Here's how the part is built. I have some questions about the finished solid (model axes, mm). A direction names the side the tool comes from. Give positions to 0.01 mm unless a question says otherwise; leave off trailing zeros. Write each loop counter-clockwise with the first axis right and the second up, starting at its lowest first coordinate (ties: lowest second). Pieces come first, ordered by that corner, then holes. Notation, with made-up numbers: M 88.25,-18.5 L 121.25,-18.5 A19 ccw 121.25,-3.5 Z; hole C 73.5,-33 d5. An arc over 180 degrees is marked long. Answer as CSV lines item,"result". Start each with the question number.
Q1. Suppose I cut it at C-C (x = -37). Write out the boundary of the cut face in (y, z).
Q2. For pin 1 (4 mm diameter, centred on x = -14.5, z = -57.5, fed in from -Y), with a flat end and sliding along its axis, tell me the tip position at first contact or that it passes through.
Q3. Thinking about a two-plate mould opening in Z: for faces 3 (the flat face through (-38, 10, -75)), 4 (the cylindrical face through (-26.508, 10.14, -40.304)), 5 (the flat face through (0, 10, -38)), which applies, +Z half, -Z half, draft (parallel to the pull), parting line (faces both ways), or undercut?
Q4. Suppose I cut it at B-B (z = -37). Write out the boundary of the cut face in (x, y).
Q5. On a 3-axis mill with a long thin cutter (end or side, diameter ignored), from which of +Z, -Z, +X, -X, +Y, -Y can I reach the whole of each face in a straight line? I mean faces 1 (the flat face through (-37, 10, 0)), 2 (the flat face through (-37, 7, -5)). Say none if no direction works.
Q6. If I drill on line 1 along Z through (x, y) = (-37, 8.5); line 2 along Z through (x, y) = (-18.5, 2), over which ranges is the centre line in solid material (lowest first)?
Q7. Suppose I cut it at A-A (y = 9.5). Write out the boundary of the cut face in (x, z), then the cut area to 3 significant figures.
Q8. Suppose I cut it at D-D (x = -64.5). Write out the boundary of the cut face in (y, z).
Autodesk Inventor part; units mm, degrees
ref_plane "YZ Plane" through (0, 0, 0) normal (1, 0, 0) x (0, 1, 0)
ref_plane "XZ Plane" through (0, 0, 0) normal (0, 1, 0) x (-1, 0, 0)
ref_plane "XY Plane" through (0, 0, 0) normal (0, 0, 1) x (1, 0, 0)
sketch "Sketch1" plane through (0, 0, 0) normal (0, 1, 0) x (-1, 0, 0)
  point P0 (0, 0)
sketch "Sketch2" plane through (0, 0, 0) normal (0, 1, 0) x (-1, 0, 0)
  line L0 (0, 0) -> (75, 0)
  line L1 (75, 0) -> (75, -75)
  line L2 (75, -75) -> (0, -75)
  line L3 (0, -75) -> (0, 0)
  dimension "d0" = 75
  dimension "d1" = 75
extrude "Extrusion1" add sketch "Sketch2" along normal blind 20
sketch "Sketch3" plane through (0, 20, 0) normal (0, 1, 0) x (1, 0, 0)
  circle A0 centre (-37, 37) radius 11
  point P0 (0, 0)
extrude "Extrusion2" cut sketch "Sketch3" against normal blind 39
shell "Shell1" thickness 5 removed faces 1 at (-37.7753, 0, -65.9733)
properties part number "B9A"
Resolved:
1,outline,"M 0,-75 L 20,-75 L 20,-48 L 0,-48 L 0,-53 L 15,-53 L 15,-70 L 0,-70 Z; M 0,-26 L 20,-26 L 20,0 L 0,0 L 0,-5 L 15,-5 L 15,-21 L 0,-21 Z"
2,pin 1,"y = 15"
3,face 3,"-Z half"
3,face 4,"undercut"
3,face 5,"draft"
4,outline,"M -75,0 L -70,0 L -70,15 L -53,15 L -53,0 L -48,0 L -48,20 L -75,20 Z; M -26,0 L -21,0 L -21,15 L -5,15 L -5,0 L 0,0 L 0,20 L -26,20 Z"
5,face 1,"+Z, +X, -X, +Y, -Y"
5,face 2,"-Y"
6,line 1,"-75 to -70, -53 to -48, -26 to -21, -5 to 0"
6,line 2,"-75 to -70, -5 to 0"
7,outline,"M -75,-75 L 0,-75 L 0,0 L -75,0 Z; C -37,-37 d32; hole M -70,-70 L -5,-70 L -5,-5 L -70,-5 Z; hole C -37,-37 d22"
7,area,"1,820 mm^2"
8,outline,"M 0,-75 L 20,-75 L 20,0 L 0,0 L 0,-5 L 15,-5 L 15,-70 L 0,-70 Z"
